Study the drawing (mm; zero at the part's minimum x, y, z) and answer. A direction names the side the tool comes from. Round coordinates to 2 decimals unless told otherwise and drop trailing zeros. Loops run counter-clockwise (first coordinate to the right, second up) from the corner with the lowest first, then second, coordinate; pieces in that order, holes last. Notation, with made-up numbers: (-37, -9.75) -> (-16, -9.75) arc R26 cw to (-16, 22.25) -> close; hole circle Ø11 at (29, 31.5). An arc over 180 degrees is marked (long way). Use one line per item in the form item = value.
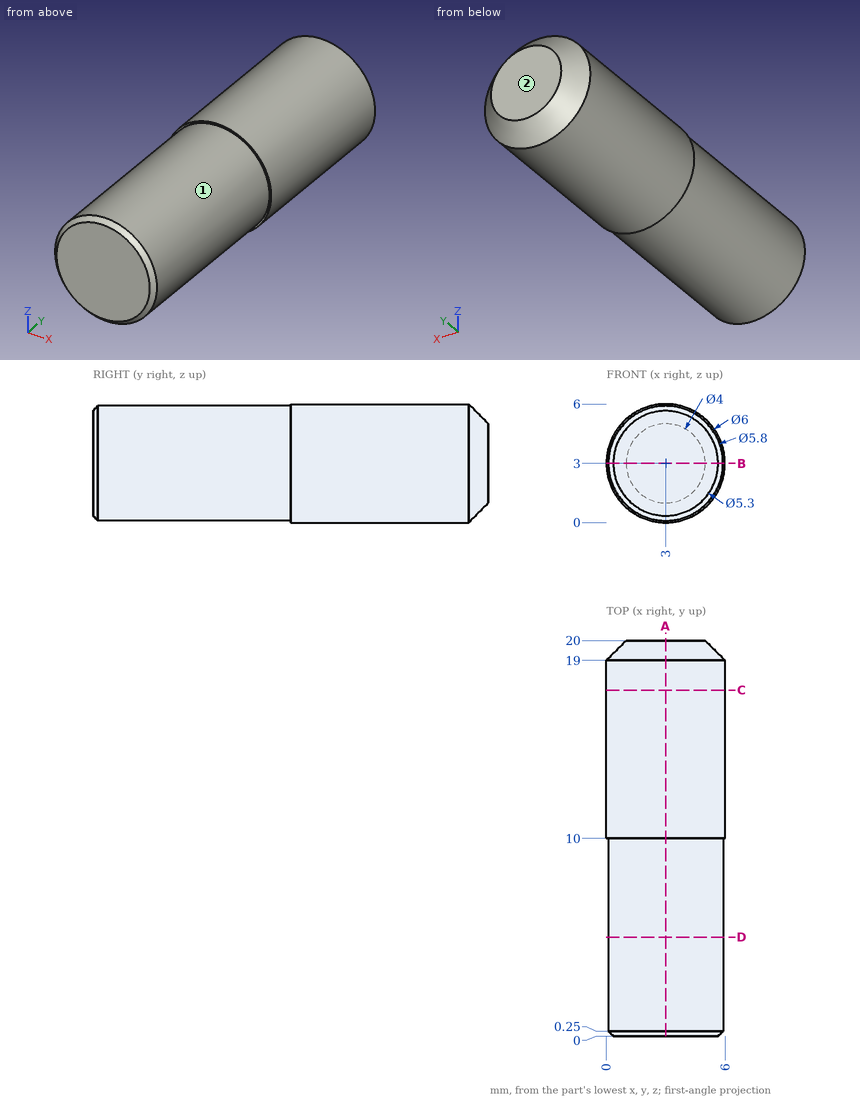
(1) Find section A-A, the plane x = 3. Write down the section's boundary in (y, z).
Completed:
outline = (0, 0.35) -> (0.25, 0.1) -> (10, 0.1) -> (10, 0) -> (19, 0) -> (20, 1) -> (20, 5) -> (19, 6) -> (10, 6) -> (10, 5.9) -> (0.25, 5.9) -> (0, 5.65) -> close
(2) Find section B-B, the plane z = 3. Write down the section's boundary in (x, y), then the cut area to 3 significant figures.
Completed:
outline = (0, 10) -> (0.1, 10) -> (0.1, 0.25) -> (0.35, 0) -> (5.65, 0) -> (5.9, 0.25) -> (5.9, 10) -> (6, 10) -> (6, 19) -> (5, 20) -> (1, 20) -> (0, 19) -> close
area = 117 mm2
(3) Find section C-C, the plane y = 17.5. Write down the section's boundary in (x, z).
Completed:
outline = circle Ø6 at (3, 3)
(4) Consider L1, parallel to X at y = 1.75, z = 3; L2, parallel to X at y = 13.25, z = 3.15; L3, parallel to Z at x = 5.3, y = 13.75. Determine where each line is inside the solid, lowest interval first.
Completed:
L1 = 0.1 to 5.9
L2 = 0 to 6
L3 = 1.07 to 4.93
(5) Given P1, Ø2, axis at x = 4, y = 2.5, coming from the -Z side, flat-ended and moving along its own axis, determine where the tip first touches the part or whether it passes through.
Completed:
P1 = 0.1
(6) For the marked faces 1 and 2, determine the directions among +Z, -Z, +X, -X, +Y, -Y from which every point of the face is accessible in a straight line to the end or side of a thin tool.
Completed:
face_1 = -Y
face_2 = +Z, -Z, +X, -X, +Y
(7) Find section D-D, the plane y = 5. Write down the section's boundary in (x, z), then the cut area to 3 significant figures.
Completed:
outline = circle Ø5.8 at (3, 3)
area = 26.4 mm2
